Input: part model. Units: mm. Frame: model coordinates. A direction names the side the tool comes from. Round coordinates to 2 decimals unless told otherwise and drop trailing zeros. Loops run counter-clockwise (first coordinate to the right, second up) from the corner with the lowest first, then second, coordinate; pieces in that order, holes last. Notation, with made-up numbers: (0.25, 86.5) -> (43.25, 86.5) arc R21 cw to (43.25, 101.5) -> close; hole circle Ø4 at (-1.75, -2). An arc over 180 degrees is marked (long way). One line per question, with ' | ' between items. Start each with the question number.
Q1. Cut plane B-B on y = 29.5. Return loops of the section in (x, z).
Q2. Cut plane D-D on z = -67. Return loops of the section in (x, y).
Q3. Mould query, pull axis Z, two halves, no side actions, for faces 1 (the face through (73.06, 9.16, -57.77)), 2 (the face through (110, 47, -50)), 3 (the face through (110.14, 46.1, -84.14)). Classes: pulls with the +Z half, pulls with the -Z half, needs draft (parallel to the pull), parting line crosses it, or undercut.
Q4. Material intervals for L1, parallel to Z at x = 110, y = 35; L2, parallel to X at y = 37.5, z = -56; L3, parallel to Y at x = 15, z = -16, sorted ascending.
Q5. Contact query for flat-ended pins moving along their axis: P1, Ø11, axis at x = 60, z = -87.96, coming from the +Y side; P2, Ø5, axis at x = 110, y = 29.5, coming from the +Z side; P3, Ø2.5, axis at x = 112, y = 30, coming from the -Z side. Output: stop coordinate, or through.
Q6. Cut plane A-A on z = -39.5. Return loops of the section in (x, y).
Q7. Access query for faces 4 (the face through (110.521, 25.534, -47.675)), 5 (the face through (100, 32, -50)), 6 (the face through (25, 5, -6)), 7 (the face through (110, 12, -75)). Directions: +Z, -Z, +X, -X, +Y, -Y. A direction counts if a zero-diameter tool reaches every point of the face in a straight line with its end or side. Return the directions, or none.
Q8. Cut plane C-C on x = 25. Return loops of the section in (y, z).
from build123d import *

# Parameters (mm, degrees)
SKETCH1_W                   = 130
SKETCH1_H                   = 100
BOSS_EXTRUDE1_DEPTH         = 12
CUT_EXTRUDE1_DEPTH          = 7
SKETCH4_W                   = 20
SKETCH4_H                   = 70
BOSS_EXTRUDE2_DEPTH         = 35
SKETCH5_W                   = 25
SKETCH5_H                   = 8
SKETCH5_W_2                 = 20
SKETCH5_H_2                 = 2
FILLET1_R                   = 5
CHAMFER1_SIZE               = 2
M8_TAPPED_HOLE1_D           = 6.8
M8_TAPPED_HOLE1_DEPTH       = 5
M8_TAPPED_HOLE1_CSINK_D     = 8.05
M8_TAPPED_HOLE1_CSINK_ANGLE = 90
M8_TAPPED_HOLE1_TIP         = 2.042926105
CUT_EXTRUDE2_REACH          = 172.614
SKETCH13_R                  = 3
FILLET2_R                   = 3
FILLET3_R                   = 5


with BuildPart() as part:
    # Sketch1 → Boss-Extrude1 (new body)
    with BuildSketch(Plane(origin=(0, 0, 0), x_dir=(1, 0, 0), z_dir=(0, 1, 0))):
        with Locations((65, 50)):
            Rectangle(SKETCH1_W, SKETCH1_H)
    extrude(amount=BOSS_EXTRUDE1_DEPTH)

    # Sketch3 → Cut-Extrude1 (cut)
    with BuildSketch(Plane(origin=(0, 12, 0), x_dir=(1, 0, 0), z_dir=(0, 1, 0))):
        with BuildLine():
            Line((10, 0), (40, 0))
            ThreePointArc((40, 0), (25, 15), (10, 0))
        make_face()
    extrude(amount=-CUT_EXTRUDE1_DEPTH, mode=Mode.SUBTRACT)

    # Sketch4 → Boss-Extrude2 (add)
    with BuildSketch(Plane(origin=(0, 12, 0), x_dir=(1, 0, 0), z_dir=(0, 1, 0))):
        with Locations((110, 50)):
            Rectangle(SKETCH4_W, SKETCH4_H)
    extrude(amount=BOSS_EXTRUDE2_DEPTH)

    # Sketch5 → Cut-Revolve1 (revolve, cut)
    with BuildSketch(Plane.ZY.offset(-110), mode=Mode.PRIVATE) as cut_revolve1_sk:
        with Locations((-72.5, 33.5)):
            Rectangle(SKETCH5_W, SKETCH5_H)
        Polygon((-60, 33.5), (-60, 29.5), (-35, 29.5), (-35, 31.5), (-35, 33.5), align=None)
        with Locations((-25, 30.5)):
            Rectangle(SKETCH5_W_2, SKETCH5_H_2)
    revolve(cut_revolve1_sk.sketch.rotate(Axis((110, 29.5, -85), (0, 0, 1)), 90), axis=Axis((110, 29.5, -85), (0, 0, 1)), mode=Mode.SUBTRACT)

    # Fillet1
    fillet1_edges = [part.edges().sort_by_distance(p)[0] for p in [
        (100, 12, -50),
        (120, 12, -50),
    ]]
    fillet(fillet1_edges, radius=FILLET1_R)

    # Chamfer1
    chamfer1_edges = [part.edges().sort_by_distance(p)[0] for p in [
        (130, 12, -50),
        (85, 12, 0),
        (65, 12, -100),
        (25, 12, -15),
        (0, 12, -50),
        (5, 12, 0),
    ]]
    chamfer(chamfer1_edges, length=CHAMFER1_SIZE)

    # M8 Tapped Hole1
    with Locations(Plane(origin=(0, 12, 0), x_dir=(1, 0, 0), z_dir=(0, 1, 0))):
        with Locations((42.923730365, 75.548416342), (60, 87.955052452), (77.076269635, 75.548416342), (70.553715035, 55.474057432), (49.446284965, 55.474057432)):
            CounterSinkHole(M8_TAPPED_HOLE1_D / 2, M8_TAPPED_HOLE1_CSINK_D / 2, depth=M8_TAPPED_HOLE1_DEPTH, counter_sink_angle=M8_TAPPED_HOLE1_CSINK_ANGLE)
            with Locations((0, 0, -(M8_TAPPED_HOLE1_DEPTH + M8_TAPPED_HOLE1_TIP / 2))):  # 118° drill point
                Cone(0, M8_TAPPED_HOLE1_D / 2, M8_TAPPED_HOLE1_TIP, mode=Mode.SUBTRACT)

    # Cut-Extrude2: up to this face of the body (flat: up to its plane)
    cut_extrude2_end = Plane(part.part.faces().sort_by_distance((56.685777118, 12, -51.176723205))[0])
    # Sketch13 → Cut-Extrude2 (cut, up to the picked face)
    with BuildSketch(Plane(origin=(0, 47, 0), x_dir=(1, 0, 0), z_dir=(0, 1, 0)), mode=Mode.PRIVATE) as cut_extrude2_sk1:
        with Locations(Location((110, 75, 0), (0, 0, 270))):
            Circle(SKETCH13_R)
    cut_extrude2_tool1 = split(extrude(cut_extrude2_sk1.sketch, amount=-CUT_EXTRUDE2_REACH, mode=Mode.PRIVATE), bisect_by=cut_extrude2_end, keep=Keep.BOTH, mode=Mode.PRIVATE)
    # Sketch13 → Cut-Extrude2 (cut, up to the picked face)
    with BuildSketch(Plane(origin=(0, 47, 0), x_dir=(1, 0, 0), z_dir=(0, 1, 0)), mode=Mode.PRIVATE) as cut_extrude2_sk2:
        with Locations(Location((110, 25, 0), (0, 0, 270))):
            Circle(SKETCH13_R)
    cut_extrude2_tool2 = split(extrude(cut_extrude2_sk2.sketch, amount=-CUT_EXTRUDE2_REACH, mode=Mode.PRIVATE), bisect_by=cut_extrude2_end, keep=Keep.BOTH, mode=Mode.PRIVATE)
    add(cut_extrude2_tool1.solids().sort_by(Axis((110, 47, -75), (0, -1, 0)))[0], mode=Mode.SUBTRACT)
    add(cut_extrude2_tool2.solids().sort_by(Axis((110, 47, -25), (0, -1, 0)))[0], mode=Mode.SUBTRACT)

    # Fillet2
    fillet2_edges = [part.edges().sort_by_distance(p)[0] for p in [
        (110, 47, -15),
        (110, 47, -85),
    ]]
    fillet(fillet2_edges, radius=FILLET2_R)

    # Fillet3
    fillet3_edges = [part.edges().sort_by_distance(p)[0] for p in [
        (130, 0, -50),
        (0, 0, -50),
    ]]
    fillet(fillet3_edges, radius=FILLET3_R)


solid = part.part
Results:
1) outline: (100, -85) -> (102, -85) -> (102, -60) -> (106, -60) -> (106, -35) -> (108, -35) -> (108, -27.24) arc R3 cw to (108, -22.76) -> (108, -15) -> (100, -15) -> close; (112, -35) -> (114, -35) -> (114, -60) -> (118, -60) -> (118, -85) -> (120, -85) -> (120, -15) -> (112, -15) -> (112, -22.76) arc R3 cw to (112, -27.24) -> close
2) outline: (0, 5) arc R5 ccw to (5, 0) -> (125, 0) arc R5 ccw to (130, 5) -> (130, 10) -> (128, 12) -> (125, 12) arc R5 cw to (120, 17) -> (120, 47) -> (100, 47) -> (100, 17) arc R5 cw to (95, 12) -> (2, 12) -> (0, 10) -> close; hole circle Ø16 at (110, 29.5)
3) face 1: undercut | face 2: needs draft | face 3: pulls with the -Z half
4) L1: -60 to -28, -22 to -15 | L2: 100 to 120 | L3: 0 to 12
5) P1: y = 12 | P2: z = -15 | P3: z = -35
6) outline: (0, 5) arc R5 ccw to (5, 0) -> (125, 0) arc R5 ccw to (130, 5) -> (130, 10) -> (128, 12) -> (125, 12) arc R5 cw to (120, 17) -> (120, 47) -> (100, 47) -> (100, 17) arc R5 cw to (95, 12) -> (2, 12) -> (0, 10) -> close; hole circle Ø8 at (110, 29.5)
7) face 4: -Z | face 5: +Z, -Z, -X, +Y | face 6: +Z, +Y | face 7: +Y
8) outline: (0, -100) -> (10, -100) -> (12, -98) -> (12, -17) -> (10, -15) -> (5, -15) -> (5, 0) -> (0, 0) -> close
